```python
from build123d import *

# Parameters (mm, degrees)
SKETCH_2_R          = 10
SKETCH_2_R_2        = 4.505
EXTRUDE_1_DEPTH     = 2.54
SKETCH_3_R          = 4.505
SKETCH_3_R_2        = 2.75
EXTRUDE_2_DEPTH     = 4.5
SKETCH_5_R          = 1.5
CUT_EXTRUDE_1_DEPTH = 2.54
SKETCH_6_R          = 2.75
SKETCH_6_R_2        = 1.5
EXTRUDE_3_DEPTH     = 1


with BuildPart() as part:
    # 草图2 → 凸台-拉伸1 (new body)
    with BuildSketch(Plane(origin=(0, 0, 0), x_dir=(1, 0, 0), z_dir=(0, 1, 0))):
        with Locations(Location((0, 0, 0), (0, 0, 270))):
            Circle(SKETCH_2_R)
        with Locations(Location((0, 0, 0), (0, 0, 270))):
            Circle(SKETCH_2_R_2, mode=Mode.SUBTRACT)
    extrude(amount=EXTRUDE_1_DEPTH)

    # 草图3 → 凸台-拉伸2 (add)
    with BuildSketch(Plane(origin=(0, 0, 0), x_dir=(1, 0, 0), z_dir=(0, 1, 0))):
        with Locations(Location((0, 0, 0), (0, 0, 270))):
            Circle(SKETCH_3_R)
        with Locations(Location((0, 0, 0), (0, 0, 270))):
            Circle(SKETCH_3_R_2, mode=Mode.SUBTRACT)
    extrude(amount=EXTRUDE_2_DEPTH)

    # 草图5 → 切除-拉伸1 (cut)
    with BuildSketch(Plane(origin=(0, 0, 0), x_dir=(1, 0, 0), z_dir=(0, 1, 0))):
        with Locations(Location((-7.249, -0.001, 0), (0, 0, 270))):
            Circle(SKETCH_5_R)
        with Locations(Location((0, 7.25, 0), (0, 0, 270))):
            Circle(SKETCH_5_R)
        with Locations(Location((7.251, 0.001, 0), (0, 0, 270))):
            Circle(SKETCH_5_R)
        with Locations(Location((0.002, -7.25, 0), (0, 0, 270))):
            Circle(SKETCH_5_R)
    extrude(amount=CUT_EXTRUDE_1_DEPTH, mode=Mode.SUBTRACT)

    # 草图6 → 凸台-拉伸3 (add)
    with BuildSketch(Plane(origin=(0, 0, 0), x_dir=(-1, 0, 0), z_dir=(0, -1, 0))):
        with Locations(Location((0, 0, 0), (0, 0, 90))):
            Circle(SKETCH_6_R)
        with Locations(Location((0, 0, 0), (0, 0, 90))):
            Circle(SKETCH_6_R_2, mode=Mode.SUBTRACT)
    extrude(amount=-EXTRUDE_3_DEPTH)


solid = part.part
```
Part model, mm, in its own coordinate system. A direction names the side the tool comes from. Round coordinates to 2 decimals unless told otherwise and drop trailing zeros. Write each loop counter-clockwise with the first axis right and the second up, starting at its lowest first coordinate (ties: lowest second). Pieces come first, ordered by that corner, then holes. Notation, with made-up numbers: (12.5, 44.5) -> (49.5, 44.5) arc R25 ccw to (49.5, 80.5) -> close; hole circle Ø6 at (-22, 25). An arc over 180 degrees is marked (long way). Return JSON: item names as keys, results as strings. Group by question number.
Q1. Which spindle directions (+Z, -Z, +X, -X, +Y, -Y) get a long thin tool onto all of the face, cutting with end or side? Do faces 1 (the cylindrical face through (-2.685, 2.726, -0.596)), 2 (the cylindrical face through (-5.76, 1.25, -0.19)). Say none if no direction does.
Q2. Saw through at A-A on z = 0. Write the cut outline in (x, y) (3 decimals), plus the area to 3 significant figures.
Q3. Saw through at D-D on y = 4.1. Write the cut outline in (x, z) (3 decimals), plus the area to 3 significant figures.
Q4. Mould opens along Z. For faces 3 (the cylindrical face through (4.467, 3.506, -0.586)), 4 (the cylindrical face through (0.07, 1.25, -8.75)), 5 (the flat face through (-2.1, 2.54, 4.3)), 6 (the cylindrical face through (0.45, 0.49, -1.43)) say: pulls with the +Z half, pulls with the -Z half, needs draft (parallel to the pull), parting line crosses it, or undercut.
Q5. Probe L1, parallel to X at y = 0.6, z = 0; L2, parallel to Y at x = 6.25, z = 5.75; L3, parallel to X at y = 0.2, z = -7.5. List the from-to ranges inside material, lowest first. Write a range as [from, to].
Q6. Saw through at B-B on x = -6. Write the cut outline in (y, z), plus the area to 3 significant figures.
Q7. Saw through at C-C on z = -7. Write the cut outline in (x, y).
Q8. Pin check, flat tips, straight feed: pin 1 (1 mm diameter, centred on y = 0.5, z = 2.5, fed in from +X); pin 2 (1 mm diameter, centred on x = 1, y = 4, fed in from +Z); pin 3 (3 mm diameter, centred on x = 8, z = -5, fed in from +Y). Stop position of each tip, or through.
Answer:
{
 "1": {"face 1": "+Y", "face 2": "+Y, -Y"},
 "2": {"outline": "(-10, 0) -> (-8.749, 0) -> (-8.749, 2.54) -> (-10, 2.54) -> close; (-5.749, 0) -> (-1.5, 0) -> (-1.5, 1) -> (-2.75, 1) -> (-2.75, 4.5) -> (-4.505, 4.5) -> (-4.505, 2.54) -> (-5.749, 2.54) -> close; (1.5, 0) -> (5.751, 0) -> (5.751, 2.54) -> (4.505, 2.54) -> (4.505, 4.5) -> (2.75, 4.5) -> (2.75, 1) -> (1.5, 1) -> close; (8.751, 0) -> (10, 0) -> (10, 2.54) -> (8.751, 2.54) -> close", "area": "31.0 mm2"},
 "3": {"outline": "circle Ø9.01 at (0, 0); hole circle Ø5.5 at (0, 0)", "area": "40.0 mm2"},
 "4": {"face 3": "parting line crosses it", "face 4": "undercut", "face 5": "needs draft", "face 6": "undercut"},
 "5": {"L1": "[-10, -8.75], [-5.75, -1.5], [1.5, 5.75], [8.75, 10]", "L2": "[0, 2.54]", "L3": "[-6.61, -1.48], [1.48, 6.61]"},
 "6": {"outline": "(0, -8) -> (2.54, -8) -> (2.54, -0.83) -> (0, -0.83) -> close; (0, 0.83) -> (2.54, 0.83) -> (2.54, 8) -> (0, 8) -> close", "area": "36.4 mm2"},
 "7": {"outline": "(-7.14, 0) -> (-1.48, 0) -> (-1.48, 2.54) -> (-7.14, 2.54) -> close; (1.48, 0) -> (7.14, 0) -> (7.14, 2.54) -> (1.48, 2.54) -> close"},
 "8": {"pin 1": "x = 9.8", "pin 2": "z = 4.48", "pin 3": "y = 2.54"}
}
